Geometry check sheet. Reference: the model listing, model coordinates, mm. Round coordinates to 2 decimals unless told otherwise and drop trailing zeros. Write each loop counter-clockwise with the first axis right and the second up, starting at its lowest first coordinate (ties: lowest second). Pieces come first, ordered by that corner, then holes. Notation, with made-up numbers: (42, 51) -> (74, 51) arc R26 ccw to (74, 65) -> close; hole circle Ø6 at (37, 45.5). An arc over 180 degrees is marked (long way). Return JSON: item names as keys, results as strings. Group by question number.
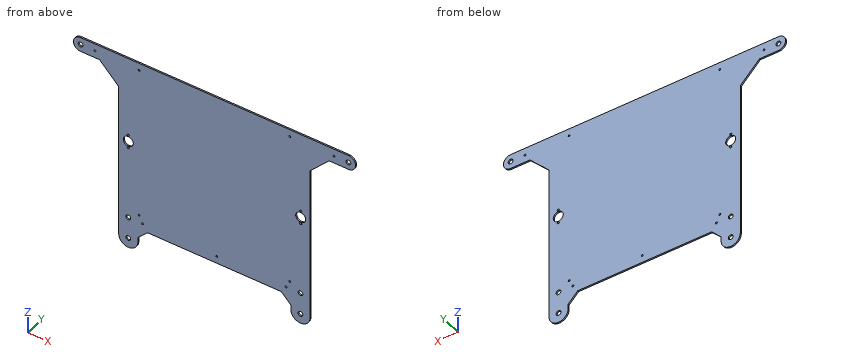
from build123d import *

# Parameters (mm, degrees)
SKETCH1_R           = 2
SKETCH1_R_2         = 5
SKETCH1_R_3         = 10.5
SKETCH1_R_4         = 2.25
BOSS_EXTRUDE1_DEPTH = 3
SKETCH2_R           = 5
BOSS_EXTRUDE2_DEPTH = 3
CHAMFER2_SIZE       = 20
CHAMFER3_SIZE       = 40


with BuildPart() as part:
    # Sketch1 → Boss-Extrude1 (new body)
    with BuildSketch(Plane(origin=(0, 0, 0), x_dir=(1, 0, 0), z_dir=(0, 1, 0))):
        with BuildLine():
            Line((-200.2851606, -142.500000035), (-280, -142.500000035))
            ThreePointArc((-280, -142.500000035), (-294.999999965, -157.5), (-280, -172.499999965))
            Line((-280, -172.499999965), (280, -172.499999965))
            ThreePointArc((280, -172.499999965), (294.999999965, -157.5), (280, -142.500000035))
            Line((280, -142.500000035), (199.7148394, -142.500000035))
            Line((199.7148394, -142.500000035), (199.7148394, 187.499999965))
            Line((199.7148394, 187.499999965), (-160.2851606, 187.499999965))
            Line((-160.2851606, 187.499999965), (-160.2851606, 217.499999965))
            ThreePointArc((-160.2851606, 217.499999965), (-180.2851606, 237.499999965), (-200.2851606, 217.499999965))
            Line((-200.2851606, 217.499999965), (-200.2851606, 187.499999965))
            Line((-200.2851606, 187.499999965), (-200.2851606, -142.500000035))
        make_face()
        with Locations(Location((-157.5, 157.5, 0), (0, 0, 270))):
            Circle(SKETCH1_R, mode=Mode.SUBTRACT)
        with Locations(Location((157.5, 157.5, 0), (0, 0, 270))):
            Circle(SKETCH1_R, mode=Mode.SUBTRACT)
        with Locations(Location((157.5, -157.5, 0), (0, 0, 270))):
            Circle(SKETCH1_R, mode=Mode.SUBTRACT)
        with Locations(Location((-157.5, -157.5, 0), (0, 0, 270))):
            Circle(SKETCH1_R, mode=Mode.SUBTRACT)
        with Locations(Location((-280, -157.5, 0), (0, 0, 270))):
            Circle(SKETCH1_R_2, mode=Mode.SUBTRACT)
        with Locations(Location((280, -157.5, 0), (0, 0, 270))):
            Circle(SKETCH1_R_2, mode=Mode.SUBTRACT)
        with Locations(Location((-250, -157.5, 0), (0, 0, 270))):
            Circle(SKETCH1_R, mode=Mode.SUBTRACT)
        with Locations(Location((250, -157.5, 0), (0, 0, 270))):
            Circle(SKETCH1_R, mode=Mode.SUBTRACT)
        with Locations(Location((-180.2851606, 172.499999965, 0), (0, 0, 270))):
            Circle(SKETCH1_R_2, mode=Mode.SUBTRACT)
        with Locations(Location((179.7148394, 172.499999965, 0), (0, 0, 270))):
            Circle(SKETCH1_R_2, mode=Mode.SUBTRACT)
        with Locations(Location((-150.2851606, 172.499999965, 0), (0, 0, 270))):
            Circle(SKETCH1_R, mode=Mode.SUBTRACT)
        with Locations(Location((4.7148394, 172.499999965, 0), (0, 0, 270))):
            Circle(SKETCH1_R, mode=Mode.SUBTRACT)
        with Locations(Location((149.7148394, 172.499999965, 0), (0, 0, 270))):
            Circle(SKETCH1_R, mode=Mode.SUBTRACT)
        with Locations(Location((-180.2851606, 7.499999983, 0), (0, 0, 270))):
            Circle(SKETCH1_R_3, mode=Mode.SUBTRACT)
        with Locations(Location((-180.2851606, 20.999999983, 0), (0, 0, 270))):
            Circle(SKETCH1_R_4, mode=Mode.SUBTRACT)
        with Locations(Location((-180.2851606, -6.000000017, 0), (0, 0, 270))):
            Circle(SKETCH1_R_4, mode=Mode.SUBTRACT)
        with Locations(Location((180.2851606, -6.000000017, 0), (0, 0, 90))):
            Circle(SKETCH1_R_4, mode=Mode.SUBTRACT)
        with Locations(Location((180.2851606, 20.999999983, 0), (0, 0, 90))):
            Circle(SKETCH1_R_4, mode=Mode.SUBTRACT)
        with Locations(Location((180.2851606, 7.499999983, 0), (0, 0, 90))):
            Circle(SKETCH1_R_3, mode=Mode.SUBTRACT)
        with Locations(Location((-180.2851606, 217.499999965, 0), (0, 0, 270))):
            Circle(SKETCH1_R_2, mode=Mode.SUBTRACT)
    extrude(amount=BOSS_EXTRUDE1_DEPTH)

    # Sketch2 → Boss-Extrude2 (add)
    with BuildSketch(Plane(origin=(0, 3, 0), x_dir=(1, 0, 0), z_dir=(0, 1, 0))):
        with BuildLine():
            Line((199.7148394, 187.499999965), (199.7148394, 217.499999965))
            ThreePointArc((199.7148394, 217.499999965), (179.7148394, 237.499999965), (159.7148394, 217.499999965))
            Line((159.7148394, 217.499999965), (159.7148394, 187.499999965))
            Line((159.7148394, 187.499999965), (199.7148394, 187.499999965))
        make_face()
        with Locations(Location((179.7148394, 217.499999965, 0), (0, 0, 270))):
            Circle(SKETCH2_R, mode=Mode.SUBTRACT)
    extrude(amount=-BOSS_EXTRUDE2_DEPTH)

    # Chamfer2
    chamfer2_edges = [part.edges().sort_by_distance(p)[0] for p in [
        (159.7148394, 1.5, -187.499999965),
        (-160.2851606, 1.5, -187.499999965),
    ]]
    chamfer(chamfer2_edges, length=CHAMFER2_SIZE)

    # Chamfer3
    chamfer3_edges = [part.edges().sort_by_distance(p)[0] for p in [
        (-200.2851606, 1.5, 142.500000035),
        (199.7148394, 1.5, 142.500000035),
    ]]
    chamfer(chamfer3_edges, length=CHAMFER3_SIZE)


solid = part.part
1) Go/stop test with flat-tipped pins: P1, Ø1.5, axis at y = 2, z = -105.5, coming from the +X side; P2, Ø0.9, axis at y = 2, z = -212.5, coming from the -X side; P3, Ø2.5, axis at x = -157.5, z = -157.5, coming from the -Y side; P4, Ø0.9, axis at x = 28, y = 2, coming from the -Z side. Record where each tip stops, or that it passes through.
2) Sectioned sample at B-B on x = 70. Enter the section's corners in (y, z), and give its area (3 significant figures).
3) Material ranges on probe 1 along X at (y, z) = (2.35, -172.5); probe 2 along X at (y, z) = (1.65, -7.5); probe 3 along Z at (x, y) = (-157.5, 1.5), recorded low to high. Write a range as [from, to].
4) Sectioned sample at C-C on z = -126. Enter the section's corners in (x, y).
5) Sectioned sample at D-D on y = 1.05. State how many separate pieces and enclosed holes the cut face has, and give its area (3 significant figures).
6) Sectioned sample at A-A on z = -200.5. Enter the section's corners in (x, y), and give its area (3 significant figures).
Evaluation:
{
 "1": {"P1": "stops at x = 199.71", "P2": "stops at x = -200.29", "P3": "passes through", "P4": "stops at z = -187.5"},
 "2": {"outline": "(0, -187.5) -> (3, -187.5) -> (3, 172.5) -> (0, 172.5) -> close", "area": "1,080 mm2"},
 "3": {"probe 1": "x = [-200.29, -185.29], [-175.29, -152.29], [-148.29, 2.71], [6.71, 147.71], [151.71, 174.71], [184.71, 199.71]", "probe 2": "x = [-200.29, -190.79], [-169.79, 169.79], [190.79, 199.71]", "probe 3": "z = [-204.71, -159.5], [-155.5, 155.5], [159.5, 172.5]"},
 "4": {"outline": "(-200.29, 0) -> (199.71, 0) -> (199.71, 3) -> (-200.29, 3) -> close"},
 "5": {"separate pieces": "1", "enclosed holes": "21", "area": "154,000 mm2"},
 "6": {"outline": "(-200.29, 0) -> (-153.29, 0) -> (-153.29, 3) -> (-200.29, 3) -> close; (152.71, 0) -> (199.71, 0) -> (199.71, 3) -> (152.71, 3) -> close", "area": "282 mm2"}
}
